Input: part model. Units: mm. Frame: model coordinates. A direction names the side the tool comes from. Give positions to 0.01 mm unless a question says otherwise; leave off trailing zeros. Write each loop counter-clockwise with the first axis right and the second up, starting at its lowest first coordinate (ties: lowest second). Pieces come first, ordered by that corner, then holes. Notation, with made-up numbers: (88.5, 53) - (104.5, 53) arc R20 ccw to (104.5, 70) - close; hole circle Ø2 at (-6.5, 46). An arc over 180 degrees is marked (long way). Answer as CSV lines item,"result". Start each with the question number.
from build123d import *

# Parameters (mm, degrees)
ESBO_O1_W                                           = 360
ESBO_O1_H                                           = 67
RESSALTO_EXTRUS_O1_DEPTH                            = 16
CORTE_EXTRUS_O1_DEPTH                               = 367.531035521
REBAIXO_PARA_PARAFUSO_COM_CABE_A_PANELA_D           = 9
REBAIXO_PARA_PARAFUSO_COM_CABE_A_PANELA_CBORE_D     = 18
REBAIXO_PARA_PARAFUSO_COM_CABE_A_PANELA_CBORE_DEPTH = 6


with BuildPart() as part:
    # Esboço1 → Ressalto-extrusão1 (new body)
    with BuildSketch(Plane.XY):
        with Locations((180, 33.5)):
            Rectangle(ESBO_O1_W, ESBO_O1_H)
    extrude(amount=RESSALTO_EXTRUS_O1_DEPTH)

    # Esboço2 → Corte-extrusão1 (cut, through all)
    with BuildSketch(Plane.ZY):
        Polygon((5, 0), (16, 25), (16, 0), align=None)
        Polygon((5, 67), (16, 42), (16, 67), align=None)
    extrude(amount=-CORTE_EXTRUS_O1_DEPTH, mode=Mode.SUBTRACT)

    # Rebaixo para parafuso com cabeça panela de M81 (through all)
    with Locations(Plane.XY.offset(16)):
        with Locations((40, 50), (40, 17), (180, 50), (180, 17), (320, 50), (320, 17)):
            CounterBoreHole(REBAIXO_PARA_PARAFUSO_COM_CABE_A_PANELA_D / 2, REBAIXO_PARA_PARAFUSO_COM_CABE_A_PANELA_CBORE_D / 2, REBAIXO_PARA_PARAFUSO_COM_CABE_A_PANELA_CBORE_DEPTH)


solid = part.part
1) Material intervals for line 1 (Y direction, x = 40, z = 3.75); line 2 (X direction, y = 50, z = 12.15); line 3 (X direction, y = 44, z = 13.75), sorted ascending. Write a range as from..to.
2) Cut plane B-B on x = 180. Output: boundary loops of the cut face in (y, z), and give its area (3 significant figures).
3) Pull-direction query (X, two-part tool) for faces 3 (the cylindrical face through (40, 41, 12)), 4 (the flat face through (360, 33, 6)), 5 (the cylindrical face through (175.708, 18.352, 4.93)), 6 (the flat face through (177, 34, 16)); classes: +X half, -X half, draft (parallel to the pull), parting line (faces both ways), or undercut.
4) Reachability of faces 1 (the flat face through (180, 45, 10)), 2 (the flat face through (0, 33, 6)) from +Z, -Z, +X, -X, +Y, -Y: full face, straight path, thin tool, end or side. Return the list, or none.
5) Contact query for flat-ended pins moving along their axis: P1, Ø8, axis at x = 189.5, y = 16.5, coming from the +Z side; P2, Ø3, axis at x = 46, z = 8, coming from the -Y side; P3, Ø7.5, axis at x = 43.5, y = 17, coming from the +Z side. Output: stop coordinate, or through.
6) Cut plane A-A on y = 50. Output: boundary loops of the cut face in (x, z).
7) Cut plane C-C on x = 295.5. Output: boundary loops of the cut face in (y, z), and give its area (3 significant figures).
Numbers:
1,line 1,"y = 0..12.5, 21.5..45.5, 54.5..67"
1,line 2,"x = 0..31, 49..171, 189..311, 329..360"
1,line 3,"x = 0..33.29, 46.71..173.29, 186.71..313.29, 326.71..360"
2,outline,"(0, 0) - (12.5, 0) - (12.5, 10) - (11.36, 10) - (0, 5) - close; (21.5, 0) - (45.5, 0) - (45.5, 10) - (41, 10) - (41, 16) - (26, 16) - (26, 10) - (21.5, 10) - close; (54.5, 0) - (67, 0) - (67, 5) - (55.64, 10) - (54.5, 10) - close"
2,area,"523 mm²"
3,face 3,"undercut"
3,face 4,"+X half"
3,face 5,"undercut"
3,face 6,"draft"
4,face 1,"+Z"
4,face 2,"+Z, -Z, -X, +Y, -Y"
5,P1,"stops at z = 14.02"
5,P2,"stops at y = 3.41"
5,P3,"stops at z = 10"
6,outline,"(0, 0) - (35.5, 0) - (35.5, 10) - (31, 10) - (31, 12.48) - (0, 12.48) - close; (44.5, 0) - (175.5, 0) - (175.5, 10) - (171, 10) - (171, 12.48) - (49, 12.48) - (49, 10) - (44.5, 10) - close; (184.5, 0) - (315.5, 0) - (315.5, 10) - (311, 10) - (311, 12.48) - (189, 12.48) - (189, 10) - (184.5, 10) - close; (324.5, 0) - (360, 0) - (360, 12.48) - (329, 12.48) - (329, 10) - (324.5, 10) - close"
7,outline,"(0, 0) - (67, 0) - (67, 5) - (42, 16) - (25, 16) - (0, 5) - close"
7,area,"797 mm²"
